CAD build for the part. Positions are in the model's coordinates, mm. Round coordinates to 2 decimals unless told otherwise and drop trailing zeros. Loops run counter-clockwise (first coordinate to the right, second up) from the corner with the lowest first, then second, coordinate; pieces in that order, holes last.
```python
from build123d import *

# Parameters (mm, degrees)
F0_W     = 457.2
F0_H     = 38.1
F0_R     = 1.984375
F1_DEPTH = 19.05
F2_SIZE  = 5.08
F3_R     = 5.08


with BuildPart() as f1:
    # F0 (on Top) → F1 (new body)
    with BuildSketch(Plane.XY):
        with Locations((228.6, 19.05)):
            Rectangle(F0_W, F0_H)
        with Locations((8.73125, 19.05)):
            Circle(F0_R, mode=Mode.SUBTRACT)
        with Locations((448.46875, 19.05)):
            Circle(F0_R, mode=Mode.SUBTRACT)
    extrude(amount=F1_DEPTH)

    # F2
    f2_edges = [f1.edges().sort_by_distance(p)[0] for p in [
        (0, 19.05, 19.05),
        (457.2, 19.05, 19.05),
    ]]
    chamfer(f2_edges, length=F2_SIZE)

    # F3
    f3_edges = [f1.edges().sort_by_distance(p)[0] for p in [
        (228.6, 38.1, 19.05),
        (228.6, 0, 19.05),
    ]]
    fillet(f3_edges, radius=F3_R)


solid = f1.part
```
Item 1: Cut at A-A, the plane x = 127. Give the cut face in (y, z), plus the area to 3 significant figures.
Answers follow:
outline: (0, 0) - (38.1, 0) - (38.1, 13.97) arc R5.08 ccw to (33.02, 19.05) - (5.08, 19.05) arc R5.08 ccw to (0, 13.97) - close
area: 715 mm2
Item 2: Probe line 1 (Y direction, x = 86.5, z = 17.5); line 2 (Y direction, x = 301.5, z = 15.25); line 3 (Z direction, x = 360.5, y = 2.5). List the from-to ranges inside material, lowest first.
Answers follow:
line 1: y = 1.43 to 36.67
line 2: y = 0.16 to 37.94
line 3: z = 0 to 18.35
Item 3: Flat gauge pins, fed straight in: P1, Ø3, axis at x = 379, y = 24.5, coming from the -Z side; P2, Ø3.5, axis at x = 8.73, y = 19.05, coming from the +Z side; P3, Ø1.5, axis at y = 15.5, z = 16.5, coming from the +X side. Where does each tip first touch, or does it go through?
Answers follow:
P1: stops at z = 0
P2: passes through
P3: stops at x = 455.42
